Check sheet for the modelled part. Datum: model origin and axes. Units: mm. Round coordinates to 2 decimals unless told otherwise and drop trailing zeros. Order: outer loops, then holes, each group sorted by start corner. A loop starts at its lowest first (then second) coordinate and runs counter-clockwise, first axis right, second up. Notation, with made-up numbers: (-18.5, 11) -> (14.5, 11) arc R25 ccw to (14.5, 29) -> close; hole circle Ø9 at (48, 9). An arc over 180 degrees is marked (long way). Answer in a Markdown table with one row per item.
Autodesk Inventor part; units mm, degrees
ref_plane "YZ Plane" through (0, 0, 0) normal (1, 0, 0) x (0, 1, 0)
ref_plane "XZ Plane" through (0, 0, 0) normal (0, 1, 0) x (-1, 0, 0)
ref_plane "XY Plane" through (0, 0, 0) normal (0, 0, 1) x (1, 0, 0)
sketch "Sketch1" plane through (0, 0, 0) normal (0, 0, 1) x (1, 0, 0)
  line L0 (-40.3138, 25.1032) -> (45.6862, 25.1032)
  line L1 (45.6862, 25.1032) -> (45.6862, -17.3968)
  line L2 (45.6862, -17.3968) -> (-40.3138, -17.3968)
  line L3 (-40.3138, -17.3968) -> (-40.3138, 25.1032)
  point P0 (0, 0)
  dimension "d0" = 86
  dimension "d1" = 42.5
extrude "Extrusion1" add sketch "Sketch1" along normal blind 2
sketch "Sketch2" plane through (0, 0, 2) normal (0, 0, 1) x (1, 0, 0)
  line L0 (-40.3138, -17.3968) -> (45.6862, -17.3968)
  line L1 (-3.3138, -17.3968) -> (8.6862, -17.3968)
  line L2 (8.6862, -17.3968) -> (8.6862, -11.3968)
  line L3 (8.6862, -11.3968) -> (-3.3138, -11.3968)
  line L4 (-3.3138, -11.3968) -> (-3.3138, -17.3968)
  line L5 (-40.3138, 25.1032) -> (-40.3138, -17.3968)
  line L6 (45.6862, -17.3968) -> (45.6862, 25.1032)
  point P0 (0, 0)
  dimension "d4" = 6
  dimension "d5" = 12
  dimension "d6" = 37
  dimension "d7" = 86
extrude "Extrusion2" cut sketch "Sketch2" against normal blind 2
fillet "Fillet1" radius 2 2 edges at (-3.3138, -11.3968, 1) (8.6862, -11.3968, 1)
sketch "Sketch3" plane through (0, 0, 2) normal (0, 0, 1) x (1, 0, 0)
  line L0 (45.6862, 25.1032) -> (-40.3138, 25.1032)
  line L1 (45.6862, -17.3968) -> (45.6862, 25.1032)
  line L2 (-40.3138, 25.1032) -> (45.6862, 25.1032)
  line L3 (45.6862, 25.1032) -> (45.6862, 23.1032)
  line L4 (45.6862, 23.1032) -> (-40.3138, 23.1032)
  line L5 (-40.3138, 23.1032) -> (-40.3138, 25.1032)
  point P0 (0, 0)
  dimension "d11" = 2
extrude "Extrusion3" cut sketch "Sketch3" against normal blind 2
sketch "Sketch4" plane through (0, 0, 2) normal (0, 0, 1) x (1, 0, 0)
  line L0 (-40.3138, 23.1032) -> (-40.3138, -17.3968)
  line L1 (-40.3138, -17.3968) -> (-3.3138, -17.3968)
  line L2 (-40.3138, 23.1032) -> (-38.3138, 23.1032)
  line L3 (-38.3138, 23.1032) -> (-38.3138, -17.3968)
  line L4 (-38.3138, -17.3968) -> (-40.3138, -17.3968)
  line L5 (-40.3138, -17.3968) -> (-40.3138, 23.1032)
  line L6 (8.6862, -17.3968) -> (45.6862, -17.3968)
  line L7 (45.6862, 23.1032) -> (43.6862, 23.1032)
  line L8 (43.6862, 23.1032) -> (43.6862, -17.3968)
  line L9 (43.6862, -17.3968) -> (45.6862, -17.3968)
  line L10 (45.6862, -17.3968) -> (45.6862, 23.1032)
  line L11 (45.6862, -17.3968) -> (45.6862, 23.1032)
  point P0 (0, 0)
  dimension "d14" = 2
  dimension "d15" = 2
extrude "Extrusion4" cut sketch "Sketch4" against normal blind 2
properties part number "front-panel"
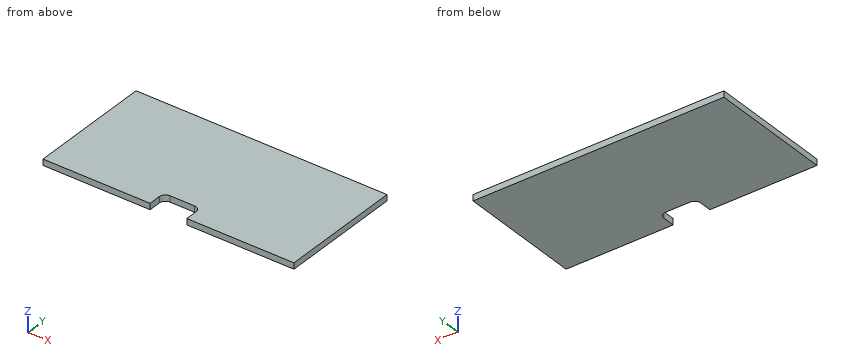
Item 1: Depth check by flat-ended pin: P1, Ø3, axis at x = -19, y = 4.5, coming from the -Z side; P2, Ø1, axis at x = -0.5, z = 1, coming from the -Y side. Enter the tip coordinate at first touch or a pass-through.
Result sheet:
| item | result |
|---|---|
| P1 | stops at z = 0 |
| P2 | stops at y = -11.4 |
Item 2: Cross-section at A-A (z = 1.55). Record the boundary of the cut face in (x, y).
Result sheet:
| item | result |
|---|---|
| outline | (-38.31, -17.4) -> (-3.31, -17.4) -> (-3.31, -13.4) arc R2 cw to (-1.31, -11.4) -> (6.69, -11.4) arc R2 cw to (8.69, -13.4) -> (8.69, -17.4) -> (43.69, -17.4) -> (43.69, 23.1) -> (-38.31, 23.1) -> close |
Item 3: Scan lines: line 1 (X direction, y = -14, z = 0.25); line 2 (Y direction, x = 7, z = 0.3). Record each from-to range of solid material in increasing order. Write a range as [from, to].
Result sheet:
| item | result |
|---|---|
| line 1 | x = [-38.31, -3.31], [8.69, 43.69] |
| line 2 | y = [-11.42, 23.1] |
Item 4: Cross-section at B-B (x = 0.5). Record the boundary of the cut face in (y, z), and give its area (3 significant figures).
Result sheet:
| item | result |
|---|---|
| outline | (-11.4, 0) -> (23.1, 0) -> (23.1, 2) -> (-11.4, 2) -> close |
| area | 69.0 mm^2 |
